Here's how the part is built. I have some questions about the finished solid (model axes, mm). A direction names the side the tool comes from. Give positions to 0.01 mm unless a question says otherwise; leave off trailing zeros. Use one line per item in the form item = value.
from build123d import *

# Parameters (mm, degrees)
SKETCH_4_R          = 11.5
EXTRUDE_1_DEPTH     = 1.5
EXTRUDE_2_DEPTH     = 4
SKETCH_7_W          = 13
SKETCH_7_H          = 10.04
CUT_EXTRUDE_3_DEPTH = 2
CUT_EXTRUDE_4_DEPTH = 38.239092514
SKETCH_9_W          = 12.301126192
SKETCH_9_H          = 2
EXTRUDE_3_DEPTH     = 1
SKETCH_10_W         = 12.301126192
SKETCH_10_H         = 2
EXTRUDE_4_DEPTH     = 1


with BuildPart() as part:
    # 草图2 → 旋转1 (revolve)
    with BuildSketch(Plane.XY):
        with BuildLine():
            Line((0, 0), (-11.5, 0))
            add(Edge.make_bspline(
                [(0, 32), (-4.710300768, 31.615095885), (-11.5, 0)],
                knots=[0, 0, 0, 1, 1, 1], degree=2, weights=[1, 2.551315819, 1]))
            Line((0, 32), (0, 0))
        make_face()
    revolve(axis=Axis((0, 0, 0), (0, 1, 0)))

    # 草图3 → 切除-旋转1 (revolve, cut)
    with BuildSketch(Plane.XY, mode=Mode.PRIVATE) as cut_revolve_1_sk:
        Polygon((0, 31), (0, 0), (-8, 0), align=None)
    revolve(cut_revolve_1_sk.sketch.rotate(Axis((0, 31, 0), (0, -1, 0)), 180), axis=Axis((0, 31, 0), (0, -1, 0)), mode=Mode.SUBTRACT)

    # 草图4 → 凸台-拉伸1 (add)
    with BuildSketch(Plane(origin=(0, 0, 0), x_dir=(1, 0, 0), z_dir=(0, 1, 0))):
        with Locations(Location((0, 0, 0), (0, 0, 270))):
            Circle(SKETCH_4_R)
    extrude(amount=-EXTRUDE_1_DEPTH)

    # 草图5 → 凸台-拉伸2 (add)
    with BuildSketch(Plane.XZ.offset(1.5)):
        Polygon((4.301126192, 6.4), (4.301126192, 5.02), (-6.5, 5.02), (-6.5, -5.02), (4.301126192, -5.02), (4.301126192, -6.4), (-6.618873808, -6.4), (-8, -6.4), (-8, 6.4), (-6.618873808, 6.4), align=None)
    extrude(amount=EXTRUDE_2_DEPTH)

    # 草图7 → 切除-拉伸3 (cut)
    with BuildSketch(Plane.XZ.offset(1.5)):
        Rectangle(SKETCH_7_W, SKETCH_7_H)
    extrude(amount=-CUT_EXTRUDE_3_DEPTH, mode=Mode.SUBTRACT)

    # 草图8 → 切除-拉伸4 (cut, through all)
    with BuildSketch(Plane(origin=(0, -1.5, 0), x_dir=(-1, 0, 0), z_dir=(0, -1, 0))):
        with BuildLine():
            Line((10.500185713, -4.69), (10.500185713, 4.69))
            ThreePointArc((10.500185713, 4.69), (11.5, 0), (10.500185713, -4.69))
        make_face()
        with BuildLine():
            Line((7.285, -8.898245614), (-7.285, -8.898245614))
            ThreePointArc((-7.285, -8.898245614), (0, -11.5), (7.285, -8.898245614))
        make_face()
        with BuildLine():
            Line((7.285, 8.898245614), (-7.285, 8.898245614))
            ThreePointArc((-7.285, 8.898245614), (0, 11.5), (7.285, 8.898245614))
        make_face()
    extrude(amount=-CUT_EXTRUDE_4_DEPTH, mode=Mode.SUBTRACT)

    # 草图9 → 凸台-拉伸3 (add)
    with BuildSketch(Plane.XY.offset(6.4)):
        with Locations((-1.849436904, -4.5)):
            Rectangle(SKETCH_9_W, SKETCH_9_H)
    extrude(amount=EXTRUDE_3_DEPTH)

    # 草图10 → 凸台-拉伸4 (add)
    with BuildSketch(Plane(origin=(0, 0, -6.4), x_dir=(-1, 0, 0), z_dir=(0, 0, -1))):
        with Locations((1.849436904, -4.5)):
            Rectangle(SKETCH_10_W, SKETCH_10_H)
    extrude(amount=EXTRUDE_4_DEPTH)


solid = part.part
(1) If I drill on probe 1 along Z at (x, y) = (5.75, -1); probe 2 along X at (y, z) = (-3, 2.75); probe 3 along X at (y, z) = (17, -0.75), over which ranges is the centre line in solid material (lowest first)?
Geometry says:
probe_1 = -8.9 to -5.02, 5.02 to 8.9
probe_2 = -8 to -6.5
probe_3 = -7.71 to -3.53, 3.53 to 7.71
(2) Thinking about a two-plate mould opening in Y: for faces 4 (the flat face through (0, -3, 5.02)), 5 (the flat face through (-2, -3.5, 7)), 6 (the flat face through (-7, -5.5, 2)), which applies, pulls with the +Y half, pulls with the -Y half, needs draft (parallel to the pull), parting line crosses it, or undercut?
Geometry says:
face_4 = needs draft
face_5 = undercut
face_6 = pulls with the -Y half
(3) For P1, Ø10, axis at x = -9, y = 17.5, coming from the +Z side; P2, Ø3, axis at y = 1.5, z = 1, coming from the -X side; P3, Ø2.5, axis at y = -4, z = -6.5, coming from the +X side; P4, Ø1, axis at x = -9, y = 16, coming from the +Z side, each with a flat end and sliding along its axis, tell me the tip position at first contact or that it passes through.
Geometry says:
P1 = 6.78
P2 = -10.5
P3 = 4.3
P4 = through
(4) For faces 1 (the flat face through (6.5, -1, 0)), 2 (the flat face through (-2, -2, 6.4)), 3 (the flat face through (-2, -4, 7.4)), which set-ups out of +Z, -Z, +X, -X, +Y, -Y let a thin tool reach every point of the face, with its end or its side?
Geometry says:
face_1 = -Y
face_2 = +Z, +X, -X
face_3 = +Z, +X, -X, -Y
